For this review, take the finished solid that the model builds, in its own axes (mm). A direction names the side the tool comes from. Round coordinates to 2 decimals unless told otherwise and drop trailing zeros. Loops run counter-clockwise (first coordinate to the right, second up) from the corner with the lowest first, then second, coordinate; pieces in that order, holes last.
1. Consider section A-A on x = 63.5. State the section outline as (y, z) points.
2. To check wall thickness, follow line 1 along Y through (x, z) = (63, -21); line 2 along X through (y, z) = (70.5, 14); line 3 along X through (y, z) = (3.5, -30.5). State the ranges of each line that lie inside material, in increasing order.
3. Consider section C-C on z = -58.5. State the section outline as (x, y) points.
4. Consider section B-B on y = 4. State the section outline as (x, z) points, then the cut area to 3 significant figures.
5. Draft analysis for pull direction Y (two halves, no side actions). For faces 3 (the flat face through (-27, -76.2, -16)), 4 (the flat face through (114.3, -1, -39)), 5 (the flat face through (-27, 76.2, -16)), 6 (the cylindrical face through (84, -15, -39)), state which applies: released by +Y, released by -Y, zero draft, split by the parting line, or undercut.
6. Consider section D-D on x = 93. State the section outline as (y, z) points.
7. Tool access review of faces 1 (the flat face through (37, -1, 0)), 2 (the flat face through (-2, -1, -76.2)): name each direction out of +Z, -Z, +X, -X, +Y, -Y from which nothing blocks a thin tool from reaching the whole face with its end or side.
8. Clearance check with flat-ended pins moving along their axes: pin 1 Ø6 at (x, y) = (35, 54) entering from +Z; pin 2 Ø10 at (y, z) = (-34, 18.5) entering from +X. State where each tip first meets the part, or that it passes through.
from build123d import *

# Parameters (mm, degrees)
F0_W     = 228.6
F0_H     = 152.4
F1_DEPTH = 76.2
F2_W     = 152.408811
F2_H     = 76.2
F3_DEPTH = 152.401
F5_D     = 50.8


with BuildPart() as f1:
    # F0 (on Front) → F1 (new body, symmetric)
    with BuildSketch(Plane.XZ):
        Rectangle(F0_W, F0_H)
    extrude(amount=F1_DEPTH, both=True)

    # F2 (on face) → F3 (cut, through all)
    with BuildSketch(Plane.XZ.offset(76.2)):
        with Locations((38.095595, 38.1)):
            Rectangle(F2_W, F2_H)
    extrude(amount=-F3_DEPTH, mode=Mode.SUBTRACT)

    # F5 (through all)
    with Locations(Plane.XY):
        with Locations((63.5, 0)):
            Hole(F5_D / 2)


solid = f1.part
Resolved:
1. outline: (-76.2, -76.2) - (-25.4, -76.2) - (-25.4, 0) - (-76.2, 0) - close; (25.4, -76.2) - (76.2, -76.2) - (76.2, 0) - (25.4, 0) - close
2. line 1: y = -76.2 to -25.4, 25.4 to 76.2
2. line 2: x = -114.3 to -38.11
2. line 3: x = -114.3 to 38.34, 88.66 to 114.3
3. outline: (-114.3, -76.2) - (114.3, -76.2) - (114.3, 76.2) - (-114.3, 76.2) - close; hole circle Ø50.8 at (63.5, 0)
4. outline: (-114.3, -76.2) - (38.42, -76.2) - (38.42, 0) - (-38.11, 0) - (-38.11, 76.2) - (-114.3, 76.2) - close; (88.58, -76.2) - (114.3, -76.2) - (114.3, 0) - (88.58, 0) - close
4. area: 19,400 mm2
5. face 3: released by -Y
5. face 4: zero draft
5. face 5: released by +Y
5. face 6: undercut
6. outline: (-76.2, -76.2) - (76.2, -76.2) - (76.2, 0) - (-76.2, 0) - close
7. face 1: +Z, +X, +Y, -Y
7. face 2: -Z, +X, -X, +Y, -Y
8. pin 1: stops at z = 0
8. pin 2: stops at x = -38.11
